The drawing under review shows one solid part. Ordinate dimensions are in mm from its lowest x, y, z. A direction names the side the tool comes from. Coordinates: 2 decimals unless noted, no trailing zeros. Loops run counter-clockwise (first coordinate to the right, second up) from the corner with the lowest first, then second, coordinate; pieces in that order, holes last.
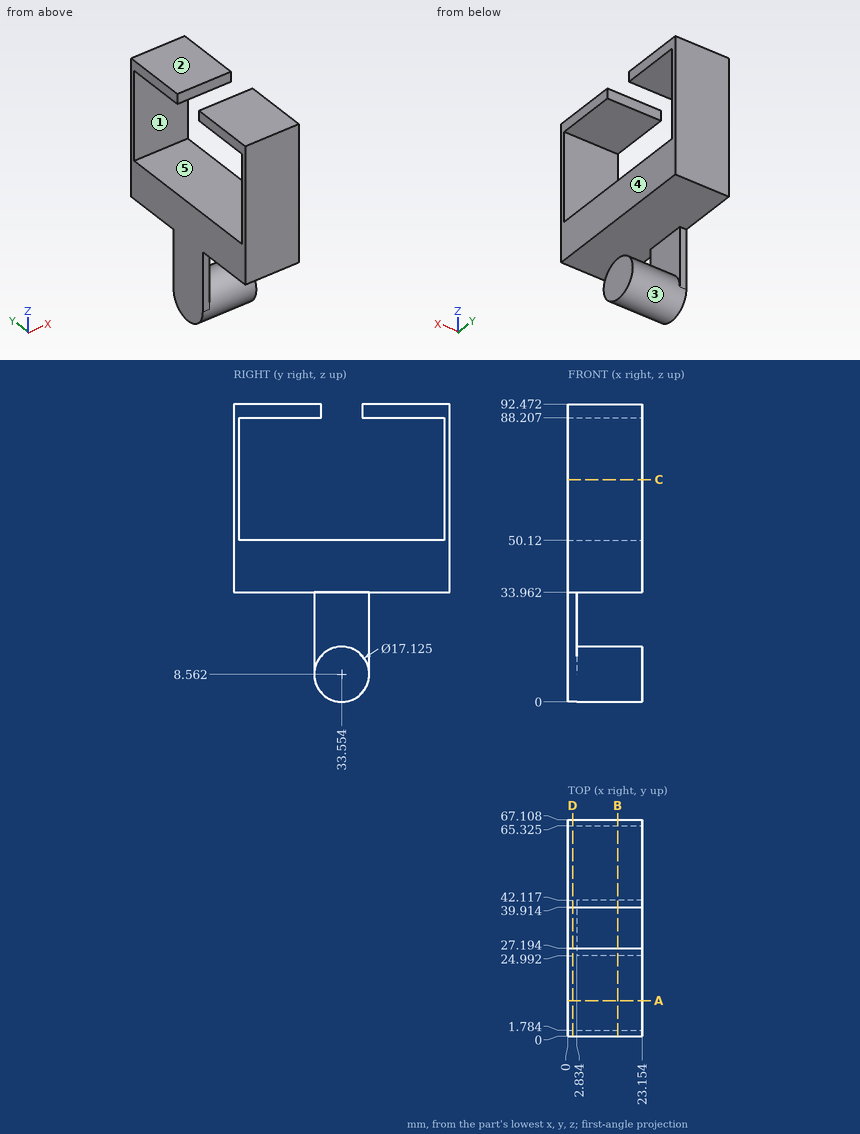
Q1. For line 1 (Z direction, x = 13.25, y = 48.5); line 2 (Y direction, x = 11, z = 74) (1 decimal); line 3 (Z direction, x = 11.25, y = 40) (1 decimal), list the stretches that pass through material, from the lowest coordinate up.
Q2. Machinability: for the marked faces 4 and 5, which of the approach directions +Z, -Z, +X, -X, +Y, -Y give a long, thin tool a straight path to every point of the face, cutting with its end or side? Answer none if there is none.
Q3. Take a section at B-B, the plane x = 15.5. Write out the cut boundary in (y, z) (1 decimal), then the cut area to 3 significant figures.
Q4. Take a section at C-C, the plane z = 69. Write out the cut boundary in (x, y) (1 decimal).
Q5. Take a section at A-A, the plane y = 11. Write out the cut boundary in (x, z).
Q6. The part is to be moulded in two halves that separate along Y. For the marked faces 1, 2 and 3, say which applies: pulls with the +Y half, pulls with the -Y half, needs draft (parallel to the pull), parting line crosses it, or undercut.
Q7. Clearance check with flat-ended pins moving along their axes: pin 1 Ø1.5 at (x, y) = (3.5, 57) entering from -Z; pin 2 Ø1.5 at (x, y) = (19.5, 27.5) entering from -Z; pin 3 Ø2.5 at (x, z) = (2, 19) entering from +Y. State where each tip first meets the part, or that it passes through.
Q8. Take a section at D-D, the plane x = 1.5. Write out the cut boundary in (y, z) (1 decimal), then the cut area to 3 significant figures.
Entries:
1. line 1: z = 33.96 to 50.12, 88.21 to 92.47
1. line 2: y = 0 to 1.8, 65.3 to 67.1
1. line 3: z = 2.9 to 14.2, 34 to 50.1, 88.2 to 92.5
2. face 4: +Z, -Z, +X, +Y, -Y
2. face 5: +X, -X
3. outline: (0, 34) - (67.1, 34) - (67.1, 92.5) - (39.9, 92.5) - (39.9, 88.2) - (65.3, 88.2) - (65.3, 50.1) - (1.8, 50.1) - (1.8, 88.2) - (27.2, 88.2) - (27.2, 92.5) - (0, 92.5) - close; circle Ø17.1 at (33.6, 8.6)
3. area: 1,680 mm2
4. outline: (0, 0) - (23.2, 0) - (23.2, 1.8) - (0, 1.8) - close; (0, 65.3) - (23.2, 65.3) - (23.2, 67.1) - (0, 67.1) - close
5. outline: (0, 33.96) - (23.15, 33.96) - (23.15, 50.12) - (0, 50.12) - close; (0, 88.21) - (23.15, 88.21) - (23.15, 92.47) - (0, 92.47) - close
6. face 1: undercut
6. face 2: needs draft
6. face 3: parting line crosses it
7. pin 1: stops at z = 33.96
7. pin 2: stops at z = 1.84
7. pin 3: stops at y = 42.12
8. outline: (0, 34) - (25, 34) - (25, 8.6) arc R8.6 ccw to (42.1, 8.6) - (42.1, 34) - (67.1, 34) - (67.1, 92.5) - (39.9, 92.5) - (39.9, 88.2) - (65.3, 88.2) - (65.3, 50.1) - (1.8, 50.1) - (1.8, 88.2) - (27.2, 88.2) - (27.2, 92.5) - (0, 92.5) - close
8. area: 2,000 mm2
